Autodesk Inventor part; units mm, degrees
ref_plane "YZ Plane" through (0, 0, 0) normal (1, 0, 0) x (0, 1, 0)
ref_plane "XZ Plane" through (0, 0, 0) normal (0, 1, 0) x (-1, 0, 0)
ref_plane "XY Plane" through (0, 0, 0) normal (0, 0, 1) x (1, 0, 0)
sketch "スケッチ1" plane through (0, 0, 0) normal (1, 0, 0) x (0, 1, 0)
  circle A0 centre (0, 0) radius 4.575
  circle A1 centre (0, 0) radius 3.575
  line L0 (0, 0) -> (0, 6)
  line L1 (0, 6) -> (0, -6)
  circle A2 centre (0, 6) radius 1.25
  circle A3 centre (0, -6) radius 1.25
  line L2 (0, 0) -> (11.5, 0)
  line L3 (11.5, 0) -> (11.5, 9.5)
  line L4 (11.5, 9.5) -> (11.5, -9.5)
  circle A4 centre (11.5, 9.5) radius 1.65
  circle A5 centre (11.5, -9.5) radius 1.65
  line L5 (0, 0) -> (0, 11.25)
  line L6 (0, 11.25) -> (0, -11.25)
  line L7 (-2.5, -11.25) -> (2.5, -11.25)
  line L8 (2.5, -11.25) -> (2.5, 11.25)
  line L9 (2.5, 11.25) -> (-2.5, 11.25)
  line L10 (-2.5, 11.25) -> (-2.5, -11.25)
  line L11 (-2.5, -11.25) -> (2.5, 11.25) construction
  line L12 (2.5, -11.25) -> (-2.5, 11.25) construction
  circle A6 centre (11.5, 9.5) radius 2.5
  circle A7 centre (11.5, -9.5) radius 2.5
  line L13 (2.5, 11.25) -> (11.2899, 11.9912)
  line L14 (2.5, -11.25) -> (11.2899, -11.9912)
  line L15 (14, 9.5) -> (14, -9.5)
  line L16 (0, -3.575) -> (14, -3.575)
  line L17 (0, 3.575) -> (14, 3.575)
  circle A8 centre (0, 0) radius 6
  line L18 (0, 0) -> (0, 6.15)
  line L19 (0, 6.15) -> (0, -6.15)
  circle A9 centre (0, 6.15) radius 1.25
  circle A10 centre (0, -6.15) radius 1.25
  point P0 (0, 7.25)
  point P1 (0, 4.75)
  point P2 (0, 4.575)
  point P3 (0, -4.575)
  point P4 (0, -4.75)
  point P5 (0, -7.25)
  point P6 (2.5, 3.575)
  point P7 (2.5, 2.5555)
  point P8 (2.5, -2.5555)
  point P9 (2.5, -3.575)
  point P10 (0, 7.4)
  point P11 (0, 4.9)
  point P12 (0, -4.9)
  point P13 (0, -7.4)
  dimension "d0" = 9.15
  dimension "d1" = 7.15
  dimension "d2" = 6
  dimension "d3" = 12
  dimension "d4" = 2.5
  dimension "d5" = 2.5
  dimension "d6" = 11.5
  dimension "d7" = 9.5
  dimension "d8" = 19
  dimension "d9" = 3.3
  dimension "d10" = 3.3
  dimension "d11" = 11.25
  dimension "d12" = 22.5
  dimension "d13" = 5
  dimension "d14" = 5
  dimension "d15" = 5
  dimension "d28" = 12
  dimension "d29" = 6.15
  dimension "d30" = 12.3
  dimension "d31" = 2.5
  dimension "d32" = 2.5
extrude "押し出し1" add sketch "スケッチ1" along normal blind 10 contours L2 A8 L16 A0 | A0 L17 A8 L2 | A0 L8 A8 L17 | L16 A8 L8 A0 | A8 L17 L3 L2 | L2 L4 L16 A8 | A0 L0 A2 A8 L8 | A8 L8 L13 A6 L3 L17 | L8 A8 A3 L1 A0 | L16 L4 A7 L14 L8 A8 | L3 L17 L15 L16 L4 | A8 A2 A9 L5 L9 L8 | L3 A6 L15 L17 | L8 L7 L6 A10 A3 A8 | L16 L15 A7 L4 | L0 A9 A8 A2 | A8 A9 A2 | A6 | A3 A8 A10 L1 | A3 A10 A8 | A7 picked at (0.1008, 4.8124) picked at (1.2329, 5.9096) picked at (0.1008, -4.8124) picked at (1.2329, -5.9096)
extrude "押し出し2" add sketch "スケッチ1" against normal blind 3 contours L2 A1 L8 L17 A0 | L2 A8 L16 A0 | A0 L16 L8 A1 L2 | A0 L17 A8 L2 | A8 L17 L3 L2 | L2 L4 L16 A8 | L3 L17 L15 L16 L4
sketch "スケッチ2" plane through (10, 0, 0) normal (1, 0, 0) x (0, 0, -1)
  circle A0 centre (0, 0) radius 3.575
  line L0 (-3.575, 14) -> (-9.5, 14)
  line L1 (-3.575, 0) -> (-3.575, 14)
  line L2 (3.575, 2.8548) -> (3.575, 14)
  line L3 (-3.575, 14) -> (3.575, 14)
  line L4 (3.575, 14) -> (3.575, 0)
  line L5 (-11.9912, 11.2899) -> (-11.25, 2.5)
  line L6 (11.25, -2.5) -> (-11.25, -2.5)
  line L7 (-11.25, -2.5) -> (-11.25, 2.5)
  line L8 (-11.25, 2.5) -> (11.25, 2.5)
  line L9 (11.25, 2.5) -> (11.25, -2.5)
  line L10 (11.25, -2.5) -> (-11.25, 2.5) construction
  line L11 (-11.25, -2.5) -> (11.25, 2.5) construction
  circle A1 centre (0, 0) radius 4.575
  point P0 (-3.575, 2.8548)
  point P1 (-3.575, 2.5)
  point P2 (-2.5555, 2.5)
  point P3 (2.5555, 2.5)
  point P4 (3.575, 2.5)
extrude "押し出し4" add sketch "スケッチ2" along normal blind 0.5 contours A1 L1 L3 L2
extrude "押し出し5" add sketch "スケッチ2" along normal blind 3 contours A0 L8 L1 A1 L4 | A1 L1 L3 L2
extrude "押し出し6" cut sketch "スケッチ2" along normal blind 0.5 contours A0 L8 L1 A1 L4
properties part number "ikafly3.3c"
Geometry: final body of the model. Coordinates: model frame, mm. A direction names the side the tool comes from. Coordinates: 2 decimals unless noted, no trailing zeros. Order: outer loops, then holes, each group sorted by start corner. A loop starts at its lowest first (then second) coordinate and runs counter-clockwise, first axis right, second up. Notation, with made-up numbers: M 22.25,22 L 72.25,22 A26 cw 72.25,58 Z; hole C 12,74 d8. An arc over 180 degrees is marked long. Answer in a Markdown table with one row per item. Add a question column.
Q1. Contact query for flat-ended pins moving along their axis: P1, Ø8, axis at x = 2.5, y = 4, coming from the -Z side; P2, Ø0.8, axis at x = -2, z = 3, coming from the -Y side; P3, Ø4, axis at x = 5, y = 3, coming from the +Z side. Output: stop coordinate, or through.
Q2. Section query A-A on z = -9. Return the cut outline in (x, y), and give its area (3 significant figures).
Q3. Section query D-D on z = -6.15. Return the cut outline in (x, y), and give its area (4 significant figures).
Q4. Section query C-C on y = 4.25. Return the cut outline in (x, z) (3 decimals), and give its area (3 significant figures).
Q5. Mould query, pull axis X, two halves, no side actions, for faces 1 (the cylindrical face through (4.93, 1.25, 6.18)), 2 (the flat face through (0, 7, -8)), 3 (the flat face through (10.5, 4, 0)). Classes: released by +X, released by -X, zero draft, split by the parting line, or undercut.
Q6. Reachability of faces 4 (the flat face through (5, 0, -9)), 5 (the flat face through (-1, 8, 3.575)), 6 (the flat face through (13, 8, 0)), 7 (the flat face through (-1, 8, -3.575)), 8 (the flat face through (11, 8, -3.575)) from +Z, -Z, +X, -X, +Y, -Y: full face, straight path, thin tool, end or side. Return the list, or none.
Q7. Line query: L1, parallel to Z at x = 4.5, y = 11.5; L2, parallel to Y at x = 6, z = -9.5; L3, parallel to Z at x = 12.75, y = 10.5 (3 decimals). Output: solid intervals per line, ascending.
Completed:
| question | item | result |
|---|---|---|
| 1 | P1 | stops at z = -11.71 |
| 1 | P2 | stops at y = 2.5 |
| 1 | P3 | stops at z = 11.46 |
| 2 | outline | M 0,0 L 10,0 L 10,9.93 L 0,9.93 Z; M 0,13.07 L 10,13.07 L 10,14 L 0,14 Z |
| 2 | area | 109 mm2 |
| 3 | outline | M 0,1.25 L 10,1.25 L 10,14 L 0,14 Z |
| 3 | area | 127.5 mm2 |
| 4 | outline | M -3,-3.575 L 0,-3.575 L 0,-11.398 L 10,-11.398 L 10,-3.575 L 13,-3.575 L 13,3.575 L 10,3.575 L 10,11.398 L 0,11.398 L 0,3.575 L -3,3.575 Z; hole M 0,-1.694 L 10.5,-1.694 L 10.5,1.694 L 0,1.694 Z |
| 4 | area | 235 mm2 |
| 5 | face 1 | zero draft |
| 5 | face 2 | released by -X |
| 5 | face 3 | undercut |
| 6 | face 4 | +Z, -Z, +X, -X, -Y |
| 6 | face 5 | +Z, -X, +Y, -Y |
| 6 | face 6 | +Z, -Z, +X, +Y, -Y |
| 6 | face 7 | -Z, -X, +Y, -Y |
| 6 | face 8 | -Z, +X, +Y, -Y |
| 7 | L1 | z = -12 to -11.15, -7.85 to 7.85, 11.15 to 12 |
| 7 | L2 | y = 0 to 9.85, 13.15 to 14 |
| 7 | L3 | z = -3.575 to 3.575 |
